Here's the drawing with two shaded views (mm, measured from the low corner). I have some questions. Give positions to 0.01 mm unless a question says otherwise; leave off trailing zeros. Loops run counter-clockwise (first coordinate to the right, second up) from the corner with the lowest first, then second, coordinate; pieces in that order, holes last. Notation, with made-up numbers: (87, 43.5) -> (93, 43.5) arc R20 cw to (93, 80.5) -> close; hole circle Ø7 at (-12, 6.25). An arc over 180 degrees is marked (long way). Answer in a Markdown table with one row per item. Add a question column.
Item 1: If we section it at A-A (y = 13.5): Write out the boundary of the cut face in (x, z), then the cut area to 3 significant figures.
Item 2: If we section it at B-B (x = 33.5): Write out the boundary of the cut face in (y, z).
Item 3: If we section it at D-D (y = 61.5): Write out the boundary of the cut face in (x, z), then the cut area to 3 significant figures.
Item 4: For P1, Ø3, axis at x = 53.5, y = 53.5, coming from the -Z side, with a flat end and sliding along its axis, tell me the tip position at first contact or that it passes through.
Item 5: If I drill on line 1 (Y direction, x = 13.5, z = 1.6); line 2 (Y direction, x = 33.5, z = 1.8); line 3 (X direction, y = 11.5, z = 1.95), over which ranges is the centre line in solid material (lowest first)?
Item 6: If we section it at C-C (z = 1.25): Write out the boundary of the cut face in (x, y).
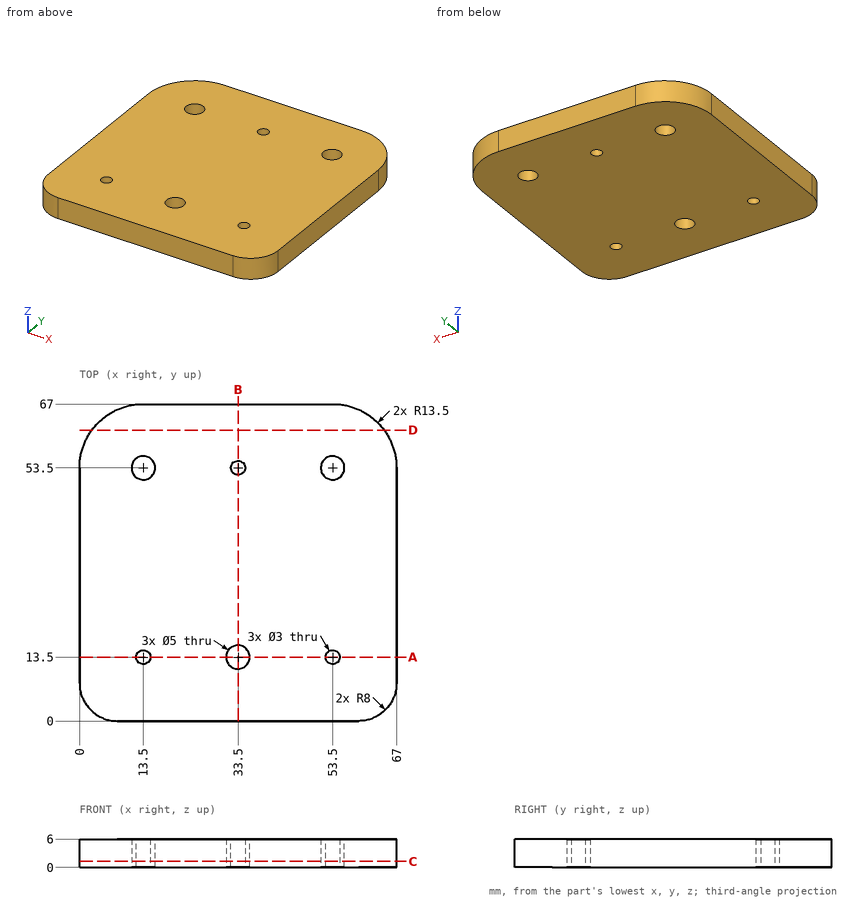
Recorded:
| question | item | result |
|---|---|---|
| 1 | outline | (0, 0) -> (12, 0) -> (12, 6) -> (0, 6) -> close; (15, 0) -> (31, 0) -> (31, 6) -> (15, 6) -> close; (36, 0) -> (52, 0) -> (52, 6) -> (36, 6) -> close; (55, 0) -> (67, 0) -> (67, 6) -> (55, 6) -> close |
| 1 | area | 336 mm^2 |
| 2 | outline | (0, 0) -> (11, 0) -> (11, 6) -> (0, 6) -> close; (16, 0) -> (52, 0) -> (52, 6) -> (16, 6) -> close; (55, 0) -> (67, 0) -> (67, 6) -> (55, 6) -> close |
| 3 | outline | (2.63, 0) -> (64.37, 0) -> (64.37, 6) -> (2.63, 6) -> close |
| 3 | area | 370 mm^2 |
| 4 | P1 | passes through |
| 5 | line 1 | y = 0 to 12, 15 to 51, 56 to 67 |
| 5 | line 2 | y = 0 to 11, 16 to 52, 55 to 67 |
| 5 | line 3 | x = 0 to 32, 35 to 67 |
| 6 | outline | (0, 8) arc R8 ccw to (8, 0) -> (59, 0) arc R8 ccw to (67, 8) -> (67, 53.5) arc R13.5 ccw to (53.5, 67) -> (13.5, 67) arc R13.5 ccw to (0, 53.5) -> close; hole circle Ø5 at (13.5, 53.5); hole circle Ø3 at (13.5, 13.5); hole circle Ø5 at (33.5, 13.5); hole circle Ø3 at (33.5, 53.5); hole circle Ø5 at (53.5, 53.5); hole circle Ø3 at (53.5, 13.5) |
